from build123d import *

# Parameters (mm, degrees)
SKETCH1_R           = 5.75
SKETCH1_R_2         = 15.75
SKETCH1_R_3         = 2
BOSS_EXTRUDE1_DEPTH = 10


with BuildPart() as part:
    # Sketch1 → Boss-Extrude1 (new body)
    with BuildSketch(Plane(origin=(0, 0, 0), x_dir=(1, 0, 0), z_dir=(0, 1, 0))):
        with BuildLine():
            Line((-104.546683395, 31), (240.453316605, 31))
            ThreePointArc((240.453316605, 31), (271.453316605, 0), (240.453316605, -31))
            Line((240.453316605, -31), (-104.546683395, -31))
            ThreePointArc((-104.546683395, -31), (-135.546683395, 0), (-104.546683395, 31))
        make_face()
        with Locations((240.453316605, 0)):
            Circle(SKETCH1_R, mode=Mode.SUBTRACT)
        with Locations((-104.546683395, 0)):
            Circle(SKETCH1_R_2, mode=Mode.SUBTRACT)
        with Locations((223.132808529, -10)):
            Circle(SKETCH1_R_3, mode=Mode.SUBTRACT)
        with Locations((223.124915417, 9.986328729)):
            Circle(SKETCH1_R_3, mode=Mode.SUBTRACT)
        with Locations((240.429637268, 19.986328729)):
            Circle(SKETCH1_R_3, mode=Mode.SUBTRACT)
        with Locations((257.742252232, 10)):
            Circle(SKETCH1_R_3, mode=Mode.SUBTRACT)
        with Locations((257.750145344, -9.986328729)):
            Circle(SKETCH1_R_3, mode=Mode.SUBTRACT)
        with Locations((240.445423493, -19.986328729)):
            Circle(SKETCH1_R_3, mode=Mode.SUBTRACT)
        with Locations((-128.046683395, 0)):
            Circle(SKETCH1_R_3, mode=Mode.SUBTRACT)
        with Locations((-116.300629951, 20.344761353)):
            Circle(SKETCH1_R_3, mode=Mode.SUBTRACT)
        with Locations((-92.808523063, 20.344761353)):
            Circle(SKETCH1_R_3, mode=Mode.SUBTRACT)
        with Locations((-81.062469619, 0)):
            Circle(SKETCH1_R_3, mode=Mode.SUBTRACT)
        with Locations((-92.808523063, -20.344761353)):
            Circle(SKETCH1_R_3, mode=Mode.SUBTRACT)
        with Locations((-116.300629951, -20.344761353)):
            Circle(SKETCH1_R_3, mode=Mode.SUBTRACT)
        with BuildLine():
            Line((-49.546683395, 15), (45.453316605, 15))
            ThreePointArc((45.453316605, 15), (60.453316605, 0), (45.453316605, -15))
            Line((45.453316605, -15), (-49.546683395, -15))
            ThreePointArc((-49.546683395, -15), (-64.546683395, 0), (-49.546683395, 15))
        make_face(mode=Mode.SUBTRACT)
        with BuildLine():
            Line((90.453316605, 15), (185.453316605, 15))
            ThreePointArc((185.453316605, 15), (200.453316605, 0), (185.453316605, -15))
            Line((185.453316605, -15), (90.453316605, -15))
            ThreePointArc((90.453316605, -15), (75.453316605, 0), (90.453316605, 15))
        make_face(mode=Mode.SUBTRACT)
    extrude(amount=BOSS_EXTRUDE1_DEPTH)


solid = part.part
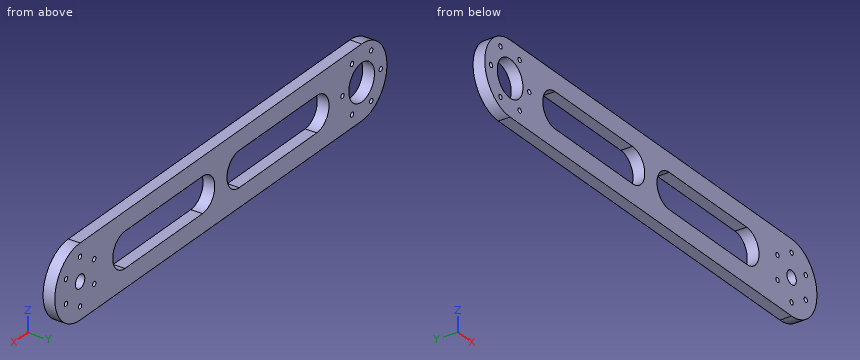
Source: CAD feature listing. Evaluate the final solid. Frame: model axes, mm. Give positions to 0.01 mm unless a question says otherwise; leave off trailing zeros. Write each loop counter-clockwise with the first axis right and the second up, starting at its lowest first coordinate (ties: lowest second). Pieces come first, ordered by that corner, then holes. Notation, with made-up numbers: M 10.25,41.5 L 51.25,41.5 A14 ccw 51.25,50.5 Z; hole C -39.75,37.25 d4. An arc over 180 degrees is marked long. Answer as a JSON object with one key per item and string values.
Q1. Cut plane D-D, the plane z = -27. Return the cut outline in (x, y), then the cut area to 3 significant figures.
Geometry check:
{"outline": "M -119.78,0 L 255.68,0 L 255.68,10 L -119.78,10 Z", "area": "3,750 mm^2"}
Q2. Ray query, line 1 along Z through (x, y) = (-12.5, 8.5); line 2 along X through (y, z) = (7, 5); line 3 along X through (y, z) = (2, -4.5). Return the intervals inside material, ascending.
Geometry check:
{"line 1": "z = -31 to -15, 15 to 31", "line 2": "x = -135.14 to -119.48, -89.61 to -63.69, 59.6 to 76.31, 199.6 to 237.61, 243.29 to 271.05", "line 3": "x = -135.22 to -119.64, -89.45 to -63.86, 59.76 to 76.14, 199.76 to 236.87, 244.03 to 271.12"}
Q3. Cut plane A-A, the plane x = -40.5. Return the cut outline in (y, z), then the cut area to 3 significant figures.
Geometry check:
{"outline": "M 0,-31 L 10,-31 L 10,-15 L 0,-15 Z; M 0,15 L 10,15 L 10,31 L 0,31 Z", "area": "320 mm^2"}
Q4. Cut plane C-C, the plane x = 196. Return the cut outline in (y, z), then the cut area to 3 significant figures.
Geometry check:
{"outline": "M 0,-31 L 10,-31 L 10,-10.67 L 0,-10.67 Z; M 0,10.67 L 10,10.67 L 10,31 L 0,31 Z", "area": "407 mm^2"}
Q5. Contact query for flat-ended pins moving along their axis: P1, Ø4, axis at y = 4.5, z = 1, coming from the +X side; P2, Ø1.5, axis at y = 8.5, z = 10, coming from the -X side; P3, Ø2, axis at y = 4, z = 7, coming from the +X side. Output: stop coordinate, or through.
Geometry check:
{"P1": "stops at x = 271.45", "P2": "stops at x = -134.13", "P3": "stops at x = 270.87"}
Q6. Cut plane B-B, the plane y = 4. Count the separate pieces of the cut face and the enclosed holes in it, then the cut area to 3 significant figures.
Geometry check:
{"separate pieces": "1", "enclosed holes": "16", "area": "16,300 mm^2"}
